Build history of the part. All positions in model axes, mm. Face numbers are marked on the shaded views. A direction names the side the tool comes from. Coordinates: 2 decimals unless noted, no trailing zeros.
Item 1: Drill centre lines: line 1 along X through (y, z) = (65, -2.25) (3 decimals); line 2 along X through (y, z) = (-42.5, 10.25). Where is each one in solid material? Low to high.
Item 2: 3-axis set-ups, long thin cutter, end or side, ignore diameter. For the marked faces 1 and 2: which of +Z, -Z, +X, -X, +Y, -Y reach the whole face in a straight line?
Item 3: Flat gauge pins, fed straight in: pin 1 (8 mm diameter, centred on x = 67.5, y = -68, fed in from +Z); pin 2 (4 mm diameter, centred on x = -98.5, y = 23.5, fed in from -Z); pin 3 (5 mm diameter, centred on y = -92.5, z = -1, fed in from +X); pin 4 (3.5 mm diameter, centred on x = -76.2, y = 57.15, fed in from -Z). Where does each tip first touch, or does it go through?
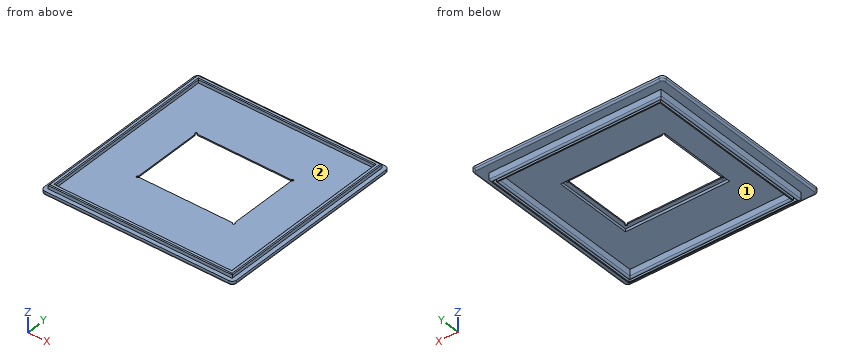
from build123d import *

# Parameters (mm, degrees)
F0_W     = 279.4
F0_H     = 279.4
F0_W_2   = 273.05
F0_H_2   = 273.05
F0_W_3   = 266.7
F0_H_3   = 266.7
F0_W_4   = 260.35
F0_H_4   = 260.35
F0_W_5   = 254
F0_H_5   = 254
F1_DEPTH = 6.35
F2_DEPTH = 12.7
F3_SIZE  = 1.27
F4_R     = 2.54
F5_DEPTH = 12.7
F6_R     = 2.54
F0_W_6   = 165.1
F0_H_6   = 127
F7_DEPTH = 6.35
F8_DEPTH = 4.445


with BuildPart() as f1:
    # F0 (on Top) → F1 (new body)
    with BuildSketch(Plane.XY):
        with BuildLine():
            Line((-139.7, -146.05), (139.7, -146.05))
            ThreePointArc((139.7, -146.05), (141.5598719395, -141.5598719395), (146.05, -139.7))
            Line((146.05, -139.7), (146.05, 139.7))
            ThreePointArc((146.05, 139.7), (141.5598719395, 141.5598719395), (139.7, 146.05))
            Line((139.7, 146.05), (-139.7, 146.05))
            ThreePointArc((-139.7, 146.05), (-141.5598719395, 141.5598719395), (-146.05, 139.7))
            Line((-146.05, 139.7), (-146.05, -139.7))
            ThreePointArc((-146.05, -139.7), (-141.5598719395, -141.5598719395), (-139.7, -146.05))
        make_face()
        Rectangle(F0_W, F0_H, mode=Mode.SUBTRACT)
        Rectangle(F0_W, F0_H)
        Rectangle(F0_W_2, F0_H_2, mode=Mode.SUBTRACT)
        Rectangle(F0_W_2, F0_H_2)
        Rectangle(F0_W_3, F0_H_3, mode=Mode.SUBTRACT)
        Rectangle(F0_W_3, F0_H_3)
        Rectangle(F0_W_4, F0_H_4, mode=Mode.SUBTRACT)
        Rectangle(F0_W_4, F0_H_4)
        Rectangle(F0_W_5, F0_H_5, mode=Mode.SUBTRACT)
        with BuildLine():
            Line((-146.049999995, -152.4), (146.05, -152.4))
            ThreePointArc((146.05, -152.4), (141.5598719395, -150.5401280605), (139.7, -146.05))
            Line((139.7, -146.05), (-139.7, -146.05))
            ThreePointArc((-139.7, -146.05), (-141.5598719377, -150.5401280588), (-146.049999995, -152.4))
        make_face()
        with BuildLine():
            ThreePointArc((139.7, 146.05), (141.5598719395, 150.5401280605), (146.05, 152.4))
            Line((146.05, 152.4), (-146.0500000019, 152.4))
            ThreePointArc((-146.0500000019, 152.4), (-141.5598719401, 150.5401280612), (-139.7, 146.05))
            Line((-139.7, 146.05), (139.7, 146.05))
        make_face()
        with BuildLine():
            ThreePointArc((146.05, -139.7), (150.5401280605, -141.5598719395), (152.4, -146.05))
            Line((152.4, -146.05), (152.4, 146.05))
            ThreePointArc((152.4, 146.05), (150.5401280605, 141.5598719395), (146.05, 139.7))
            Line((146.05, 139.7), (146.05, -139.7))
        make_face()
        with BuildLine():
            Line((-152.4, 146.0500002439), (-152.4, -146.05))
            ThreePointArc((-152.4, -146.05), (-150.5401280605, -141.5598719395), (-146.05, -139.7))
            Line((-146.05, -139.7), (-146.05, 139.7))
            ThreePointArc((-146.05, 139.7), (-150.5401281468, 141.5598720257), (-152.4, 146.0500002439))
        make_face()
        with BuildLine():
            ThreePointArc((139.7, -146.05), (141.5598719395, -150.5401280605), (146.05, -152.4))
            ThreePointArc((146.05, -152.4), (150.5401280605, -150.5401280605), (152.4, -146.05))
            ThreePointArc((152.4, -146.05), (150.5401280605, -141.5598719395), (146.05, -139.7))
            Line((146.05, -139.7), (146.05, -146.05))
            Line((146.05, -146.05), (139.7, -146.05))
        make_face()
        with BuildLine():
            ThreePointArc((-152.4, -146.05), (-150.5401280588, -150.5401280623), (-146.049999995, -152.4))
            ThreePointArc((-146.049999995, -152.4), (-141.5598719377, -150.5401280588), (-139.7, -146.05))
            Line((-139.7, -146.05), (-146.05, -146.05))
            Line((-146.05, -146.05), (-146.05, -139.7))
            ThreePointArc((-146.05, -139.7), (-150.5401280605, -141.5598719395), (-152.4, -146.05))
        make_face()
        with BuildLine():
            ThreePointArc((146.05, 139.7), (150.5401280605, 141.5598719395), (152.4, 146.05))
            ThreePointArc((152.4, 146.05), (150.5401280605, 150.5401280605), (146.05, 152.4))
            ThreePointArc((146.05, 152.4), (141.5598719395, 150.5401280605), (139.7, 146.05))
            Line((139.7, 146.05), (146.05, 146.05))
            Line((146.05, 146.05), (146.05, 139.7))
        make_face()
        with BuildLine():
            ThreePointArc((-146.0500000019, 152.4), (-150.540127975, 150.5401281461), (-152.4, 146.0500002439))
            ThreePointArc((-152.4, 146.0500002439), (-150.5401281468, 141.5598720257), (-146.05, 139.7))
            Line((-146.05, 139.7), (-146.05, 146.05))
            Line((-146.05, 146.05), (-139.7, 146.05))
            ThreePointArc((-139.7, 146.05), (-141.5598719401, 150.5401280612), (-146.0500000019, 152.4))
        make_face()
        with BuildLine():
            Line((-146.05, -146.05), (-139.7, -146.05))
            ThreePointArc((-139.7, -146.05), (-141.5598719395, -141.5598719395), (-146.05, -139.7))
            Line((-146.05, -139.7), (-146.05, -146.05))
        make_face()
        with BuildLine():
            ThreePointArc((139.7, 146.05), (141.5598719395, 141.5598719395), (146.05, 139.7))
            Line((146.05, 139.7), (146.05, 146.05))
            Line((146.05, 146.05), (139.7, 146.05))
        make_face()
        with BuildLine():
            Line((-146.05, 146.05), (-146.05, 139.7))
            ThreePointArc((-146.05, 139.7), (-141.5598719395, 141.5598719395), (-139.7, 146.05))
            Line((-139.7, 146.05), (-146.05, 146.05))
        make_face()
        with BuildLine():
            ThreePointArc((146.05, -139.7), (141.5598719395, -141.5598719395), (139.7, -146.05))
            Line((139.7, -146.05), (146.05, -146.05))
            Line((146.05, -146.05), (146.05, -139.7))
        make_face()
    extrude(amount=F1_DEPTH)

    # F0 (on Top) → F2 (join)
    with BuildSketch(Plane.XY):
        with BuildLine():
            Line((-139.7, -146.05), (139.7, -146.05))
            ThreePointArc((139.7, -146.05), (141.5598719395, -141.5598719395), (146.05, -139.7))
            Line((146.05, -139.7), (146.05, 139.7))
            ThreePointArc((146.05, 139.7), (141.5598719395, 141.5598719395), (139.7, 146.05))
            Line((139.7, 146.05), (-139.7, 146.05))
            ThreePointArc((-139.7, 146.05), (-141.5598719395, 141.5598719395), (-146.05, 139.7))
            Line((-146.05, 139.7), (-146.05, -139.7))
            ThreePointArc((-146.05, -139.7), (-141.5598719395, -141.5598719395), (-139.7, -146.05))
        make_face()
        Rectangle(F0_W, F0_H, mode=Mode.SUBTRACT)
        with BuildLine():
            Line((-146.05, 146.05), (-146.05, 139.7))
            ThreePointArc((-146.05, 139.7), (-141.5598719395, 141.5598719395), (-139.7, 146.05))
            Line((-139.7, 146.05), (-146.05, 146.05))
        make_face()
        with BuildLine():
            Line((-146.05, -146.05), (-139.7, -146.05))
            ThreePointArc((-139.7, -146.05), (-141.5598719395, -141.5598719395), (-146.05, -139.7))
            Line((-146.05, -139.7), (-146.05, -146.05))
        make_face()
        with BuildLine():
            ThreePointArc((146.05, -139.7), (141.5598719395, -141.5598719395), (139.7, -146.05))
            Line((139.7, -146.05), (146.05, -146.05))
            Line((146.05, -146.05), (146.05, -139.7))
        make_face()
        with BuildLine():
            ThreePointArc((139.7, 146.05), (141.5598719395, 141.5598719395), (146.05, 139.7))
            Line((146.05, 139.7), (146.05, 146.05))
            Line((146.05, 146.05), (139.7, 146.05))
        make_face()
    extrude(amount=F2_DEPTH)

    # F3
    f3_edges = [f1.edges().sort_by_distance(p)[0] for p in [
        (146.05, 0, 12.7),
        (139.7, 0, 12.7),
        (0, 139.7, 12.7),
        (0, 146.05, 12.7),
        (-139.7, 0, 12.7),
        (-146.05, 0, 12.7),
        (0, -139.7, 12.7),
        (0, -146.05, 12.7),
    ]]
    chamfer(f3_edges, length=F3_SIZE)

    # F4
    f4_edges = [f1.edges().sort_by_distance(p)[0] for p in [
        (0, -152.4, 0),
        (-152.4, 0, 0),
        (-150.540128, -150.540128, 0),
        (152.4, 0, 0),
        (150.540128, -150.540128, 0),
        (0, 152.4, 0),
        (-150.540128, 150.540128, 0),
        (150.540128, 150.540128, 0),
    ]]
    fillet(f4_edges, radius=F4_R)

    # F0 (on Top) → F5 (join)
    with BuildSketch(Plane.XY):
        Rectangle(F0_W_2, F0_H_2)
        Rectangle(F0_W_3, F0_H_3, mode=Mode.SUBTRACT)
        Rectangle(F0_W_4, F0_H_4)
        Rectangle(F0_W_5, F0_H_5, mode=Mode.SUBTRACT)
    extrude(amount=-F5_DEPTH)

    # F6
    f6_edges = [f1.edges().sort_by_distance(p)[0] for p in [
        (0, 136.525, -12.7),
        (-136.525, 0, -12.7),
        (0, -136.525, -12.7),
        (136.525, 0, -12.7),
        (0, 127, -12.7),
        (-127, 0, -12.7),
        (0, -127, -12.7),
        (127, 0, -12.7),
    ]]
    fillet(f6_edges, radius=F6_R)

    # F0 (on Top) → F7 (join)
    with BuildSketch(Plane.XY):
        Rectangle(F0_W_5, F0_H_5)
        Rectangle(F0_W_6, F0_H_6, mode=Mode.SUBTRACT)
        Rectangle(F0_W_6, F0_H_6)
        with BuildLine():
            ThreePointArc((-76.2, 55.245), (-77.5470384182, 58.4970384182), (-74.295, 57.15))
            Line((-74.295, 57.15), (74.295, 57.15))
            ThreePointArc((74.295, 57.15), (76.2, 59.055), (78.105, 57.15))
            ThreePointArc((78.105, 57.15), (77.5470384182, 55.8029615818), (76.2, 55.245))
            Line((76.2, 55.245), (76.2, -55.245))
            ThreePointArc((76.2, -55.245), (77.5470384182, -55.8029615818), (78.105, -57.15))
            ThreePointArc((78.105, -57.15), (76.2, -59.055), (74.295, -57.15))
            Line((74.295, -57.15), (-74.295, -57.15))
            ThreePointArc((-74.295, -57.15), (-77.5470384182, -58.4970384182), (-76.2, -55.245))
            Line((-76.2, -55.245), (-76.2, 55.245))
        make_face(mode=Mode.SUBTRACT)
    extrude(amount=F7_DEPTH)

    # F0 (on Top) → F8 (cut)
    with BuildSketch(Plane.XY):
        Rectangle(F0_W_6, F0_H_6)
        with BuildLine():
            ThreePointArc((-76.2, 55.245), (-77.5470384182, 58.4970384182), (-74.295, 57.15))
            Line((-74.295, 57.15), (74.295, 57.15))
            ThreePointArc((74.295, 57.15), (76.2, 59.055), (78.105, 57.15))
            ThreePointArc((78.105, 57.15), (77.5470384182, 55.8029615818), (76.2, 55.245))
            Line((76.2, 55.245), (76.2, -55.245))
            ThreePointArc((76.2, -55.245), (77.5470384182, -55.8029615818), (78.105, -57.15))
            ThreePointArc((78.105, -57.15), (76.2, -59.055), (74.295, -57.15))
            Line((74.295, -57.15), (-74.295, -57.15))
            ThreePointArc((-74.295, -57.15), (-77.5470384182, -58.4970384182), (-76.2, -55.245))
            Line((-76.2, -55.245), (-76.2, 55.245))
        make_face(mode=Mode.SUBTRACT)
    extrude(amount=F8_DEPTH, mode=Mode.SUBTRACT)


solid = f1.part
Filled sheet:
1. line 1: x = -136.525 to -133.35, -130.175 to -127, 127 to 130.175, 133.35 to 136.525
1. line 2: x = -146.05 to -139.7, 139.7 to 146.05
2. face 1: -Z
2. face 2: +Z
3. pin 1: stops at z = 6.35
3. pin 2: stops at z = 0
3. pin 3: stops at x = 152.18
3. pin 4: passes through
